from build123d import *

# Parameters (mm, degrees)
SKETCH1_R           = 7
BOSS_EXTRUDE1_DEPTH = 1
BOSS_EXTRUDE2_DEPTH = 1
CIRPATTERN1_COUNT   = 24


with BuildPart() as part:
    # Sketch1 → Boss-Extrude1 (new body)
    with BuildSketch(Plane.XY):
        Circle(SKETCH1_R)
    extrude(amount=BOSS_EXTRUDE1_DEPTH)

    # Sketch2 → Boss-Extrude2 (add)
    with BuildSketch(Plane.XY):
        Polygon((0, 6.72), (-0.730154643, 6.72), (-0.28, 8.4), (0.28, 8.4), (0.730154643, 6.72), align=None)
    boss_extrude2 = extrude(amount=BOSS_EXTRUDE2_DEPTH)

    # CirPattern1: Boss-Extrude2 ×24 about axis
    cirpattern1_axis = Axis((0, 0, 0), (0, 0, 1))
    for i in range(1, CIRPATTERN1_COUNT):
        add(boss_extrude2.rotate(cirpattern1_axis, i * 360 / CIRPATTERN1_COUNT))


solid = part.part
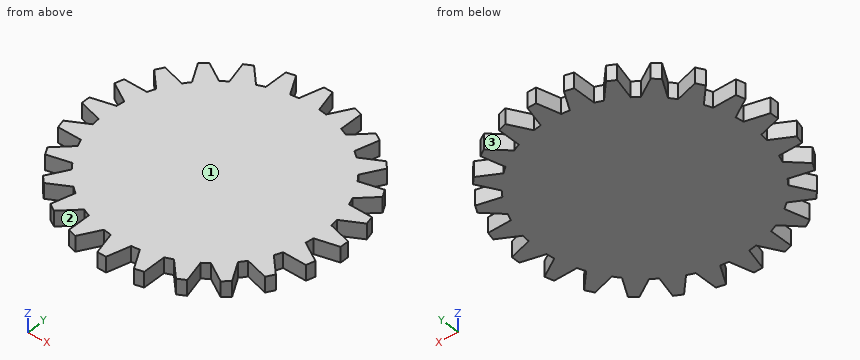
Geometry: final body of the model. Coordinates: model frame, mm. Face numbers are marked on the shaded views. Coordinates: 2 decimals unless noted, no trailing zeros. Loops run counter-clockwise (first coordinate to the right, second up) from the corner with the lowest first, then second, coordinate; pieces in that order, holes last. Notation, with made-up numbers: (3.5, -29.75) - (8.5, -29.75) arc R19 ccw to (8.5, -12.75) - close; hole circle Ø3 at (25.5, 9). An arc over 180 degrees is marked (long way). Put each result on its own line as item: value. Start each with the question number.
Q1. Cut plane A-A, the plane y = 1.5. Return loops of the section in (x, z).
Q2. Cut plane B-B, the plane x = -2.25. Return loops of the section in (y, z).
Q3. Pull-direction query (X, two-part tool) for the marked faces 1, 2 and 3; classes: released by +X, released by -X, zero draft, split by the parting line, or undercut.
Q4. Pin query (flat end, axial travel): pin 1 Ø0.5 at (x, z) = (-7.5, 0.5) entering from -Y. Return the tip coordinate at first contact, or that it passes through.
Q5. Line query: line 1 (Y direction, x = 6, z = 0.5); line 2 (Y direction, x = -7.5, z = 0.4); line 3 (X direction, y = 7.75, z = 0.5). Output: solid intervals per line, ascending.
Filled sheet:
1. outline: (-7.49, 0) - (7.49, 0) - (7.49, 1) - (-7.49, 1) - close
2. outline: (-8.09, 0) - (8.09, 0) - (8.09, 1) - (-8.09, 1) - close
3. face 1: zero draft
3. face 2: undercut
3. face 3: undercut
4. pin 1: y = -4.24
5. line 1: -5.88 to -5.5, -4.14 to 4.14, 5.5 to 5.88
5. line 2: -2.44 to -1.51, -0.52 to 0.52, 1.51 to 2.44
5. line 3: -2.44 to -1.65, -0.45 to 0.45, 1.65 to 2.44
